Autodesk Inventor part; units mm, degrees
ref_plane "YZ Plane" through (0, 0, 0) normal (1, 0, 0) x (0, 1, 0)
ref_plane "XZ Plane" through (0, 0, 0) normal (0, 1, 0) x (-1, 0, 0)
ref_plane "XY Plane" through (0, 0, 0) normal (0, 0, 1) x (1, 0, 0)
sketch "Sketch1" plane through (0, 0, 0) normal (0, 0, 1) x (1, 0, 0)
  line L0 (0, 12) -> (0, -9)
  line L1 (-9, 0) -> (12, 0)
  circle A0 centre (0, 0) radius 7.5
  dimension "d0" = 15
extrude "Extrusion1" add sketch "Sketch1" along normal blind 66
sketch "Sketch2" plane through (0, 0, 0) normal (1, 0, 0) x (0, 1, 0)
  line L0 (-3, -8.1335) -> (3, -8.1335)
  line L1 (3, -8.1335) -> (3, 18)
  line L2 (3, 18) -> (-3, 18)
  line L3 (-3, 18) -> (-3, -8.1335)
  line L4 (0, 88.24) -> (0, -15.5468)
  line L5 (-7.5, 0) -> (7.5, 0)
  dimension "d3" = 6
  dimension "d7" = 18
extrude "Extrusion2" cut sketch "Sketch2" along normal through all both and the other way through all
sketch "Sketch3" plane through (0, 0, 0) normal (0, 1, 0) x (-1, 0, 0)
  line L0 (0, -6.6) -> (0, 85.8)
  circle A0 centre (0, 8) radius 4
  line L1 (-6.8739, 0) -> (6.8739, 0)
  dimension "d8" = 8
  dimension "d9" = 8
extrude "Extrusion3" cut sketch "Sketch3" along normal through all both and the other way through all
chamfer "Chamfer1" distance 2 angle 45 2 edges at (0, -7.5, 0) (0, 7.5, 0)
chamfer "Chamfer2" distance 1 angle 45 1 edges at (-7.5, 0, 66)
hole "Hole1" at (0, 0, 66) direction (0, 0, -1) diameter 6.917 depth 30 tip angle 118
properties part number "Pin Pressure"
Input: part model. Units: mm. Frame: model coordinates. A direction names the side the tool comes from. Coordinates: 2 decimals unless noted, no trailing zeros. Loops run counter-clockwise (first coordinate to the right, second up) from the corner with the lowest first, then second, coordinate; pieces in that order, holes last.
Q1. Mould query, pull axis Y, two halves, no side actions, for faces 4 (the flat face through (0, 0, 18)), 5 (the conical face through (-0.1, -5.8, 0.3)), 6 (the flat face through (0, 4, 0)). Classes: +Y half, -Y half, draft (parallel to the pull), parting line (faces both ways), or undercut.
Results are:
face 4: undercut
face 5: -Y half
face 6: draft
Q2. Set-up query: faces 1 (the flat face through (-3, -3, 11)), 2 (the flat face through (0, -4, 0)), 3 (the cylindrical face through (-3.43, 0.45, 50.79)). Return all of +Z, -Z, +X, -X, +Y, -Y with unobstructed straight access to the full face (end or side cutting, diameter ignored); none if empty.
Results are:
face 1: -Z, +X, -X
face 2: -Z, +X, -X, +Y, -Y
face 3: +Z
Q3. Section A-A, the plane z = 14.5. Return the cut outline in (x, y), and give its area (3 significant figures).
Results are:
outline: (-6.87, -3) arc R7.5 ccw to (6.87, -3) - close; (-6.87, 3) - (6.87, 3) arc R7.5 ccw to start
area: 89.2 mm2
Q4. Section C-C, the plane x = 1.75. Give the number of separate pieces and of enclosed holes in the cut face, and give its area (3 significant figures).
Results are:
separate pieces: 3
enclosed holes: 0
area: 605 mm2
Q5. Contact query for flat-ended pins moving along their axis: pin 1 (1.5 mm diameter, centred on x = 2.5, y = 1.5, fed in from -Z); pin 2 (8 mm diameter, centred on x = -4, y = -2, fed in from -Z); pin 3 (2 mm diameter, centred on y = -3, z = 47, fed in from -X); pin 4 (1 mm diameter, centred on y = 3, z = 14, fed in from -X). Output: stop coordinate, or through.
Results are:
pin 1: stops at z = 18
pin 2: stops at z = 0
pin 3: stops at x = -7.23
pin 4: stops at x = -6.87
Q6. Section B-B, the plane z = 45. Return the cut outline in (x, y).
Results are:
outline: circle Ø15 at (0, 0); hole circle Ø6.92 at (0, 0)
Q7. Line query: line 1 along X through (y, z) = (0, 38); line 2 along Z through (x, y) = (-1, -3.25). Output: solid intervals per line, ascending.
Results are:
line 1: x = -7.5 to -3.46, 3.46 to 7.5
line 2: z = 0 to 4.13, 11.87 to 35.97
